Can you work these out from the model? Positions are in its coordinate system, mm. Round coordinates to 2 decimals unless told otherwise and drop trailing zeros. Order: outer loops, then holes, each group sorted by start corner. A loop starts at its lowest first (then second) coordinate and runs counter-clockwise, first axis right, second up.
Q1. If I drill on line 1 (X direction, y = 22, z = 1.75); line 2 (X direction, y = 21.5, z = 0.75); line 3 (Y direction, x = 355.6, z = 3), over which ranges is the centre line in solid material (lowest first)?
Q2. We'd pull the mould along Y, two halves only. Please class faces 1 (the face through (369.43, 27.22, 3.22)), 2 (the face through (206.045, 63.734, 3.131)), 3 (the face through (200, 33, 0)): pulls with the +Y half, pulls with the -Y half, needs draft (parallel to the pull), parting line crosses it, or undercut.
Q3. If we section it at B-B (y = 22.86): Please give me the cut outline in (x, z), plus the area to 3 significant figures.
Q4. If we section it at C-C (z = 3): Please give me the cut outline in (x, y), plus the area to 3 significant figures.
Q5. If we section it at D-D (y = 51): Please give me the cut outline in (x, z).
Q6. Will these pins go through, and if not, where does the flat tip stop? P1, Ø1, axis at x = 154, z = 3.5, coming from the +Y side; P2, Ø8, axis at x = 221.5, y = 64, coming from the +Z side; P3, Ø3, axis at x = 78.5, z = 2, coming from the +Y side.
Q7. If we section it at A-A (x = 363.5): Please give me the cut outline in (y, z), plus the area to 3 significant figures.
from build123d import *

# Parameters (mm, degrees)
BOSS_EXTRUDE1_DEPTH = 6.35
SKETCH2_R           = 14.499971
CUT_EXTRUDE1_DEPTH  = 6.35


with BuildPart() as part:
    # Sketch1 → Boss-Extrude1 (new body)
    with BuildSketch(Plane.XY):
        Polygon((0, 0), (406.4, 0), (406.4, 44.45), (0, 83.566), align=None)
    extrude(amount=BOSS_EXTRUDE1_DEPTH)

    # Sketch2 → Cut-Extrude1 (cut)
    with BuildSketch(Plane.XY.offset(6.35)):
        with Locations((355.6, 22.86)):
            Circle(SKETCH2_R)
    extrude(amount=-CUT_EXTRUDE1_DEPTH, mode=Mode.SUBTRACT)


solid = part.part
Solution:
1. line 1: x = 0 to 341.13, 370.07 to 406.4
1. line 2: x = 0 to 341.16, 370.04 to 406.4
1. line 3: y = 0 to 8.36, 37.36 to 49.34
2. face 1: undercut
2. face 2: pulls with the +Y half
2. face 3: needs draft
3. outline: (0, 0) - (341.1, 0) - (341.1, 6.35) - (0, 6.35) - close; (370.1, 0) - (406.4, 0) - (406.4, 6.35) - (370.1, 6.35) - close
3. area: 2,400 mm2
4. outline: (0, 0) - (406.4, 0) - (406.4, 44.45) - (0, 83.57) - close; hole circle Ø29 at (355.6, 22.86)
4. area: 25,400 mm2
5. outline: (0, 0) - (338.35, 0) - (338.35, 6.35) - (0, 6.35) - close
6. P1: stops at y = 68.79
6. P2: stops at z = 6.35
6. P3: stops at y = 76.15
7. outline: (0, 0) - (10.7, 0) - (10.7, 6.35) - (0, 6.35) - close; (35.02, 0) - (48.58, 0) - (48.58, 6.35) - (35.02, 6.35) - close
7. area: 154 mm2
